Could you check a few things on this model? Use its own coordinates, in mm. A direction names the side the tool comes from. Round coordinates to 2 decimals unless told otherwise and drop trailing zeros. Loops run counter-clockwise (first coordinate to the right, second up) from the corner with the lowest first, then second, coordinate; pieces in that order, holes last. Notation, with made-up numbers: (-16.5, 33) -> (2.5, 33) arc R35 cw to (2.5, 66) -> close; hole circle Ø7 at (49.25, 44). An arc over 180 degrees is marked (long way). One line per item, written item: value.
```python
from build123d import *

# Parameters (mm, degrees)
BOSS_EXTRUDE1_START = 2
SKETCH1_R           = 97.5
SKETCH1_R_2         = 31
SKETCH1_R_3         = 4.5
SKETCH1_R_4         = 2
BOSS_EXTRUDE1_DEPTH = 10
BOSS_EXTRUDE2_DEPTH = 2
SKETCH7_R           = 2
CUT_EXTRUDE1_DEPTH  = 10
SKETCH8_R           = 5
BOSS_EXTRUDE3_DEPTH = 12.5


with BuildPart() as part:
    # Sketch1 → Boss-Extrude1 (new body)
    with BuildSketch(Plane(origin=(0, 0, 0), x_dir=(0, 0, -1), z_dir=(1, 0, 0)).offset(BOSS_EXTRUDE1_START)):
        Circle(SKETCH1_R)
        Circle(SKETCH1_R_2, mode=Mode.SUBTRACT)
        with Locations((23.65, 31.8556608)):
            Circle(SKETCH1_R_3, mode=Mode.SUBTRACT)
        with Locations((23.932849605, -31.643709245)):
            Circle(SKETCH1_R_3, mode=Mode.SUBTRACT)
        with Locations((-23.932849605, -31.643709245)):
            Circle(SKETCH1_R_3, mode=Mode.SUBTRACT)
        with Locations((-23.65, 31.8556608)):
            Circle(SKETCH1_R_3, mode=Mode.SUBTRACT)
        with Locations((0, 80)):
            Circle(SKETCH1_R_4, mode=Mode.SUBTRACT)
        with Locations((69.282032303, -40)):
            Circle(SKETCH1_R_4, mode=Mode.SUBTRACT)
        with Locations((-69.282032303, -40)):
            Circle(SKETCH1_R_4, mode=Mode.SUBTRACT)
    extrude(amount=BOSS_EXTRUDE1_DEPTH)

    # Sketch6 → Boss-Extrude2 (add)
    with BuildSketch(Plane.ZY.offset(-2)):
        with BuildLine():
            ThreePointArc((80.491911572, 59.338454408), (70.710678119, 70.710678119), (59.338454408, 80.491911572))
            ThreePointArc((59.338454408, 80.491911572), (60.104076401, 60.104076401), (80.491911572, 59.338454408))
        make_face()
        with BuildLine():
            ThreePointArc((98.875, 14.957753006), (85, 0), (98.875, -14.957753006))
            ThreePointArc((98.875, -14.957753006), (100, 0), (98.875, 14.957753006))
        make_face()
        with BuildLine():
            ThreePointArc((80.491911572, -59.338454408), (60.104076401, -60.104076401), (59.338454408, -80.491911572))
            ThreePointArc((59.338454408, -80.491911572), (70.710678119, -70.710678119), (80.491911572, -59.338454408))
        make_face()
        with BuildLine():
            ThreePointArc((-59.338454408, -80.491911572), (-60.104076401, -60.104076401), (-80.491911572, -59.338454408))
            ThreePointArc((-80.491911572, -59.338454408), (-70.710678119, -70.710678119), (-59.338454408, -80.491911572))
        make_face()
        with BuildLine():
            ThreePointArc((-98.875, -14.957753006), (-85, 0), (-98.875, 14.957753006))
            ThreePointArc((-98.875, 14.957753006), (-100, 0), (-98.875, -14.957753006))
        make_face()
        with BuildLine():
            ThreePointArc((-80.491911572, 59.338454408), (-60.104076401, 60.104076401), (-59.338454408, 80.491911572))
            ThreePointArc((-59.338454408, 80.491911572), (-70.710678119, 70.710678119), (-80.491911572, 59.338454408))
        make_face()
    extrude(amount=BOSS_EXTRUDE2_DEPTH)

    # Sketch7 → Cut-Extrude1 (cut)
    with BuildSketch(Plane.ZY.offset(-2)):
        with Locations((0, 67)):
            Circle(SKETCH7_R)
    extrude(amount=-CUT_EXTRUDE1_DEPTH, mode=Mode.SUBTRACT)

    # Sketch8 → Boss-Extrude3 (add, symmetric)
    with BuildSketch(Plane.XY):
        with BuildLine():
            Line((-21, -60.5), (3.212451129, -60.5))
            Line((3.212451129, -60.5), (3.212451129, -71.5))
            Line((3.212451129, -71.5), (-21, -71.5))
            ThreePointArc((-21, -71.5), (-26.5, -66), (-21, -60.5))
        make_face()
        with Locations((-21, -66)):
            Circle(SKETCH8_R, mode=Mode.SUBTRACT)
    extrude(amount=BOSS_EXTRUDE3_DEPTH, both=True)


solid = part.part
```
(1) On a 3-axis mill with a long thin cutter (end or side, diameter ignored), from which of +Z, -Z, +X, -X, +Y, -Y can I reach the whole of each face in a straight line? I mean faces 1 (the face through (1.014, -59.884, 60.328)), 2 (the face through (6.93, -59.33, 77.37)), 3 (the face through (0, 66, -66)), 4 (the face through (6.93, -28.6, -20.62)). Say none if no direction works.
Results below:
face 1: -X
face 2: +X
face 3: +Z, -Z, -X, +Y, -Y
face 4: +X, -X
(2) Please list where these lines run through material, in increasing order: L1, parallel to Y at x = 4.5, z = 0; L2, parallel to Z at x = -6.5, y = -68.5; L3, parallel to X at y = 54, z = 40.
Results below:
L1: y = -97.5 to -31, 31 to 65, 69 to 78, 82 to 97.5
L2: z = -12.5 to 12.5
L3: x = 2 to 12
(3) Imagine slicing it at B-B on z = -23.65. Write out the boundary of the cut face in (x, y).
Results below:
outline: (2, -94.59) -> (12, -94.59) -> (12, -36.13) -> (2, -36.13) -> close; (2, -27.15) -> (12, -27.15) -> (12, -20.04) -> (2, -20.04) -> close; (2, 20.04) -> (12, 20.04) -> (12, 27.36) -> (2, 27.36) -> close; (2, 36.36) -> (12, 36.36) -> (12, 94.59) -> (2, 94.59) -> close
(4) For pin 1 Ø25 at (y, z) = (-66.5, -71.5) entering from +X; pin 2 Ø8 at (x, y) = (1, -6.5) entering from -Z; pin 3 Ø7.5 at (y, z) = (66.5, -65) entering from -X; pin 4 Ø1 at (y, z) = (-60.5, 20.5) entering from -X, each with a flat end and sliding along its axis, tell me the tip position at first contact or that it passes through.
Results below:
pin 1: stops at x = 12
pin 2: stops at z = -99.97
pin 3: stops at x = 0
pin 4: stops at x = 2
(5) Imagine slicing it at D-D on y = -75.5. Write out the boundary of the cut face in (x, z), then the cut area to 3 significant figures.
Results below:
outline: (0, -65.57) -> (2, -65.57) -> (2, -61.69) -> (12, -61.69) -> (12, 61.69) -> (2, 61.69) -> (2, 65.57) -> (0, 65.57) -> (0, 56.5) -> (2, 56.5) -> (2, -56.5) -> (0, -56.5) -> close
area: 1,270 mm²
(6) Imagine slicing it at A-A on y = 0. Write out the boundary of the cut face in (x, z).
Results below:
outline: (0, -100) -> (2, -100) -> (2, -97.5) -> (12, -97.5) -> (12, -31) -> (2, -31) -> (2, -85) -> (0, -85) -> close; (0, 85) -> (2, 85) -> (2, 31) -> (12, 31) -> (12, 97.5) -> (2, 97.5) -> (2, 100) -> (0, 100) -> close
(7) Imagine slicing it at C-C on x = -18.5. Write out the boundary of the cut face in (y, z), then the cut area to 3 significant figures.
Results below:
outline: (-71.5, -12.5) -> (-70.33, -12.5) -> (-70.33, 12.5) -> (-71.5, 12.5) -> close; (-61.67, -12.5) -> (-60.5, -12.5) -> (-60.5, 12.5) -> (-61.67, 12.5) -> close
area: 58.5 mm²
(8) We'd pull the mould along Y, two halves only. Please class faces 5 (the face through (1.014, 60.328, 59.884)), 6 (the face through (1.01, 70.56, 70.86)), 7 (the face through (0, -65, -66)), 8 (the face through (1.014, 59.884, -60.328)): +Y half, -Y half, draft (parallel to the pull), parting line (faces both ways), or undercut.
Results below:
face 5: undercut
face 6: +Y half
face 7: draft
face 8: undercut
